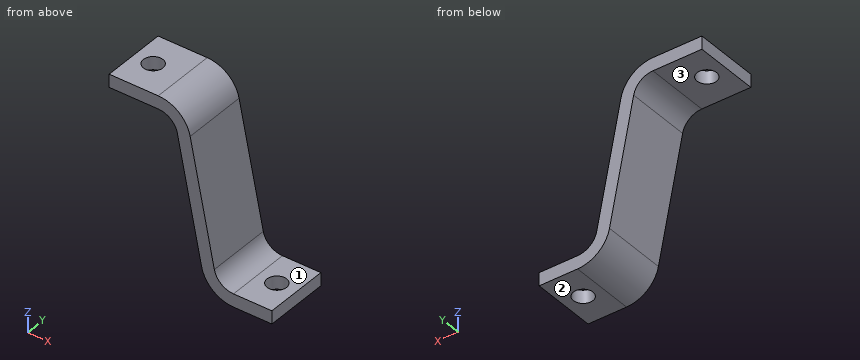
from build123d import *

# Parameters (mm, degrees)
SM_BASE_FLANGE_1_DEPTH = 10
SKETCH_9_R             = 1.5
CUT_EXTRUDE_1_DEPTH    = 10
SKETCH_10_R            = 1.5
CUT_EXTRUDE_2_DEPTH    = 10


# Sheet-metal steps are written as plain solids
with BuildPart() as part:
    # 草图4 → 基体-法兰1 (new body)
    with BuildSketch(Plane(origin=(0, 0, 0), x_dir=(1, 0, 0), z_dir=(0, 1, 0))):
        with BuildLine():
            Line((-57.778209212, -22.439021502), (-50.237620921, -22.439021502))
            ThreePointArc((-50.237620921, -22.439021502), (-48.335654204, -21.759047926), (-47.295878894, -20.027369908))
            Line((-47.295878894, -20.027369908), (-43.582093077, -1.458440827))
            ThreePointArc((-43.582093077, -1.458440827), (-41.849134227, 1.427689204), (-38.679189699, 2.560978498))
            Line((-38.679189699, 2.560978498), (-32.778209212, 2.560978498))
            Line((-32.778209212, 2.560978498), (-32.778209212, 0.560978498))
            Line((-32.778209212, 0.560978498), (-38.679189699, 0.560978498))
            ThreePointArc((-38.679189699, 0.560978498), (-40.581156416, -0.118995078), (-41.620931726, -1.850673097))
            Line((-41.620931726, -1.850673097), (-45.334717542, -20.419602178))
            ThreePointArc((-45.334717542, -20.419602178), (-47.067676393, -23.305732209), (-50.237620921, -24.439021502))
            Line((-50.237620921, -24.439021502), (-57.778209212, -24.439021502))
            Line((-57.778209212, -24.439021502), (-57.778209212, -22.439021502))
        make_face()
    extrude(amount=SM_BASE_FLANGE_1_DEPTH)

    # 草图9 → 切除-拉伸1 (cut)
    with BuildSketch(Plane(origin=(0, 0, 22.439021502), x_dir=(-1, 0, 0), z_dir=(0, 0, -1))):
        with Locations((54.778209212, 5)):
            Circle(SKETCH_9_R)
    extrude(amount=-CUT_EXTRUDE_1_DEPTH, mode=Mode.SUBTRACT)

    # 草图10 → 切除-拉伸2 (cut)
    with BuildSketch(Plane.XY.offset(-0.560978498)):
        with Locations((-35.778209212, 5)):
            Circle(SKETCH_10_R)
    extrude(amount=-CUT_EXTRUDE_2_DEPTH, mode=Mode.SUBTRACT)


solid = part.part
Build history of the part. All positions in model axes, mm. Face numbers are marked on the shaded views. A direction names the side the tool comes from. Give positions to 0.01 mm unless a question says otherwise; leave off trailing zeros. Write each loop counter-clockwise with the first axis right and the second up, starting at its lowest first coordinate (ties: lowest second). Pieces come first, ordered by that corner, then holes. Notation, with made-up numbers: (-12.5, -19) - (-1.5, -19) arc R16 ccw to (-1.5, 6) - close; hole circle Ø3 at (-37.75, 76). An arc over 180 degrees is marked (long way). Use one line per item in the form item = value. Start each with the question number.
1. 3-axis set-ups, long thin cutter, end or side, ignore diameter. For the marked faces 1, 2 and 3: which of +Z, -Z, +X, -X, +Y, -Y reach the whole face in a straight line?
2. Band-saw the part on B-B on y = 9.25. Write the cut outline in (x, z), plus the area to 3 significant figures.
3. Drop flat-ended pins along their axis: pin 1 Ø3.5 at (x, y) = (-35.78, 5) entering from +Z; pin 2 Ø2.5 at (x, y) = (-54.78, 5) entering from +Z; pin 3 Ø4 at (x, y) = (-38, 1.5) entering from +Z. Give the stop position or say it passes through.
4. Probe line 1 (Z direction, x = -35.75, y = 8.25); line 2 (X direction, y = 6, z = 22.5); line 3 (Z direction, x = -39.75, y = 6). List the from-to ranges inside material, lowest first. Write a range as [from, to].
5. Band-saw the part on D-D on z = 16.75. Write the cut outline in (x, y), plus the area to 3 significant figures.
6. Band-saw the part on C-C on z = 0.75. Write the cut outline in (x, y).
7. Band-saw the part on A-A on y = 5. Write the cut outline in (x, z), plus the area to 3 significant figures.
Conclusion:
q1.face_1 = +Z, +X, +Y, -Y
q1.face_2 = -Z, +X, -X, +Y, -Y
q1.face_3 = -Z, -X, +Y, -Y
q2.outline = (-57.78, 22.44) - (-50.24, 22.44) arc R3 cw to (-47.3, 20.03) - (-43.58, 1.46) arc R5 ccw to (-38.68, -2.56) - (-32.78, -2.56) - (-32.78, -0.56) - (-38.68, -0.56) arc R3 cw to (-41.62, 1.85) - (-45.33, 20.42) arc R5 ccw to (-50.24, 24.44) - (-57.78, 24.44) - close
q2.area = 86.7 mm²
q3.pin_1 = -0.56
q3.pin_2 = through
q3.pin_3 = -0.25
q4.line_1 = [-2.56, -0.56]
q4.line_2 = [-57.78, -55.9], [-53.66, -46.28]
q4.line_3 = [-2.44, -0.36]
q5.outline = (-46.64, 0) - (-44.6, 0) - (-44.6, 10) - (-46.64, 10) - close
q5.area = 20.4 mm²
q6.outline = (-43.39, 0) - (-41.16, 0) - (-41.16, 10) - (-43.39, 10) - close
q7.outline = (-57.78, 22.44) - (-56.28, 22.44) - (-56.28, 24.44) - (-57.78, 24.44) - close; (-53.28, 22.44) - (-50.24, 22.44) arc R3 cw to (-47.3, 20.03) - (-43.58, 1.46) arc R5 ccw to (-38.68, -2.56) - (-37.28, -2.56) - (-37.28, -0.56) - (-38.68, -0.56) arc R3 cw to (-41.62, 1.85) - (-45.33, 20.42) arc R5 ccw to (-50.24, 24.44) - (-53.28, 24.44) - close; (-34.28, -2.56) - (-32.78, -2.56) - (-32.78, -0.56) - (-34.28, -0.56) - close
q7.area = 74.7 mm²
